For this review, take the finished solid that the model builds, in its own axes (mm). A direction names the side the tool comes from. Round coordinates to 2 decimals unless told otherwise and drop trailing zeros. Write each loop counter-clockwise with the first axis right and the second up, starting at its lowest first coordinate (ties: lowest second). Pieces come first, ordered by that corner, then holes. Notation, with made-up numbers: (-29.5, -22) - (27.5, -22) arc R22 ccw to (27.5, 3) - close; hole circle Ø11 at (-26, -30.5). An arc over 180 degrees is marked (long way). One line per item, written item: value. Start each with the question number.
Q1. Add section B-B on x = 6.35. Write out the cut boundary in (y, z) (3 decimals).
Q2. Mouldability with a two-part tool opening along X and no side actions: class faces 1 (the face through (25.4, -2, -6)), 2 (the face through (20.74, -2.17, -4.52)), 3 (the face through (20.26, 0.59, -2.92)), 4 (the face through (8, -3.175, -5)) as +X half, -X half, draft (parallel to the pull), parting line (faces both ways), or undercut.
Q3. Clearance check with flat-ended pins moving along their axes: pin 1 Ø1.3 at (x, z) = (22, -9.5) entering from -Y; pin 2 Ø5 at (x, z) = (6.5, -9.5) entering from -Y (3 decimals); pin 3 Ø0.5 at (x, z) = (9.5, -9.5) entering from -Y. State where each tip first meets the part, or that it passes through.
Q4. For probe 1 along Z at (x, y) = (22.25, -0.65); probe 2 along Z at (x, y) = (6.5, -1.95); probe 3 along Z at (x, y) = (10, -2.65), list the stretches that pass through material, from the lowest coordinate up.
Q5. Add section A-A on y = -2.3. Write out the cut boundary in (x, z), and give its area (3 significant figures).
Q6. Add section C-C on y = 0.3. Write out the cut boundary in (x, z) (3 decimals).
Q7. Tool access review of faces 5 (the face through (16, 1.194, -3)), 6 (the face through (7.56, 0.59, -9.27)), 7 (the face through (13, -1.194, -6)): name each direction out of +Z, -Z, +X, -X, +Y, -Y from which nothing blocks a thin tool from reaching the whole face with its end or side.
```python
from build123d import *

# Parameters (mm, degrees)
SKETCH2_W            = 25.4
SKETCH2_H            = 12.7
BOSS_EXTRUDE1_DEPTH  = 3.175
SKETCH2_3_R          = 1.9812
BOSS_EXTRUDE2_DEPTH  = 1.1938
LPATTERN1_COUNT      = 4
LPATTERN1_PITCH      = 6.35
LPATTERN1_COUNT_DIR2 = 2
LPATTERN1_PITCH_DIR2 = 6.35
SHELL1_T             = -1.1938
SKETCH4_R            = 2.5019
SKETCH4_R_2          = 1.9812
BOSS_EXTRUDE3_DEPTH  = 1.9812
FILLET1_R            = 1.1938
FILLET2_R            = 1.1938
LPATTERN2_COUNT      = 3
LPATTERN2_PITCH      = 6.35


with BuildPart() as part:
    # Sketch2 → Boss-Extrude1 (new body)
    with BuildSketch(Plane(origin=(0, 0, 0), x_dir=(1, 0, 0), z_dir=(0, 1, 0))):
        with Locations((12.7, 6.35)):
            Rectangle(SKETCH2_W, SKETCH2_H)
    extrude(amount=-BOSS_EXTRUDE1_DEPTH)

    # Sketch2<3> → Boss-Extrude2 (add)
    with BuildSketch(Plane(origin=(0, 0, 0), x_dir=(1, 0, 0), z_dir=(0, 1, 0))):
        with Locations(Location((3.175, 9.525, 0), (0, 0, 90))):
            Circle(SKETCH2_3_R)
    boss_extrude2 = extrude(amount=BOSS_EXTRUDE2_DEPTH)

    # LPattern1: Boss-Extrude2 4 × 2
    with Locations(*[(i * LPATTERN1_PITCH, 0, j * LPATTERN1_PITCH_DIR2) for i in range(LPATTERN1_COUNT) for j in range(LPATTERN1_COUNT_DIR2) if (i, j) != (0, 0)]):
        add(boss_extrude2)

    # Shell1
    shell1_openings = [part.faces().sort_by_distance(p)[0] for p in [
        (12.7, -3.175, -6.35),
    ]]
    offset(amount=SHELL1_T, openings=shell1_openings, kind=Kind.INTERSECTION)

    # Sketch4 → Boss-Extrude3 (add)
    with BuildSketch(Plane.XZ.offset(1.1938)):
        with Locations(Location((6.35, -6.363913067, 0), (0, 0, 270))):
            Circle(SKETCH4_R)
        with Locations(Location((6.35, -6.363913067, 0), (0, 0, 270))):
            Circle(SKETCH4_R_2, mode=Mode.SUBTRACT)
    boss_extrude3 = extrude(amount=BOSS_EXTRUDE3_DEPTH)

    # Fillet1
    fillet1_edges = [part.edges().sort_by_distance(p)[0] for p in [
        (1.1938, -2.1844, -1.1938),
    ]]
    fillet(fillet1_edges, radius=FILLET1_R)

    # Fillet2
    fillet2_edges = [part.edges().sort_by_distance(p)[0] for p in [
        (1.1938, -2.1844, -11.5062),
        (24.2062, -2.1844, -11.5062),
        (24.2062, -2.1844, -1.1938),
    ]]
    fillet(fillet2_edges, radius=FILLET2_R)

    # LPattern2: Boss-Extrude3 ×3
    with Locations(*[(i * LPATTERN2_PITCH, 0, 0) for i in range(1, LPATTERN2_COUNT)]):
        add(boss_extrude3)


solid = part.part
```
Result set:
1. outline: (-3.175, -12.7) - (0, -12.7) - (0, 0) - (-3.175, 0) - (-3.175, -1.194) - (-1.194, -1.194) - (-1.194, -3.862) - (-3.175, -3.862) - (-3.175, -4.383) - (-1.194, -4.383) - (-1.194, -8.345) - (-3.175, -8.345) - (-3.175, -8.866) - (-1.194, -8.866) - (-1.194, -11.506) - (-3.175, -11.506) - close
2. face 1: +X half
2. face 2: undercut
2. face 3: undercut
2. face 4: draft
3. pin 1: stops at y = -1.19
3. pin 2: stops at y = -3.175
3. pin 3: stops at y = 0
4. probe 1: z = -12.7 to -10.31, -8.74 to -3.96, -2.39 to 0
4. probe 2: z = -12.7 to -11.51, -8.86 to -8.34, -4.39 to -3.87, -1.19 to 0
4. probe 3: z = -12.7 to -11.51, -1.19 to 0
5. outline: (0, -12.7) - (25.4, -12.7) - (25.4, 0) - (0, 0) - close; circle Ø5 at (6.35, -6.36); circle Ø5 at (12.7, -6.36); circle Ø5 at (19.05, -6.36); hole (1.19, -10.31) arc R1.19 ccw to (2.39, -11.51) - (23.01, -11.51) arc R1.19 ccw to (24.21, -10.31) - (24.21, -2.39) arc R1.19 ccw to (23.01, -1.19) - (2.39, -1.19) arc R1.19 ccw to (1.19, -2.39) - close; hole circle Ø3.96 at (6.35, -6.36); hole circle Ø3.96 at (12.7, -6.36); hole circle Ø3.96 at (19.05, -6.36)
5. area: 108 mm^2
6. outline: circle Ø3.962 at (3.175, -9.525); circle Ø3.962 at (3.175, -3.175); circle Ø3.962 at (9.525, -9.525); circle Ø3.962 at (9.525, -3.175); circle Ø3.962 at (15.875, -9.525); circle Ø3.962 at (15.875, -3.175); circle Ø3.962 at (22.225, -9.525); circle Ø3.962 at (22.225, -3.175)
7. face 5: +Z, -Z, +X, -X, +Y
7. face 6: +Y
7. face 7: -Y
